from build123d import *

# Parameters (mm, degrees)
SKETCH5_R            = 22.5
BOSS_EXTRUDE4_DEPTH  = 45
SKETCH6_R            = 21
BOSS_EXTRUDE5_DEPTH  = 6
SKETCH7_R            = 22.25
BOSS_EXTRUDE6_DEPTH  = 38
SKETCH8_R            = 21
BOSS_EXTRUDE7_DEPTH  = 22
SKETCH9_R            = 18.5
BOSS_EXTRUDE9_DEPTH  = 22
CUT_EXTRUDE1_START   = -6.5
CUT_EXTRUDE1_DEPTH   = 6.5
CUT_EXTRUDE3_START   = -38
CUT_EXTRUDE3_DEPTH   = 38
BOSS_EXTRUDE11_DEPTH = 2
SKETCH19_R           = 5
BOSS_EXTRUDE12_DEPTH = 25
CUT_EXTRUDE4_DEPTH   = 10


with BuildPart() as part:
    # Sketch5 → Boss-Extrude4 (new body)
    with BuildSketch(Plane(origin=(0, 0, 0), x_dir=(1, 0, 0), z_dir=(0, 1, 0))):
        with Locations(Location((0, 0, 0), (0, 0, 90))):
            Circle(SKETCH5_R)
    extrude(amount=BOSS_EXTRUDE4_DEPTH)

    # Sketch6 → Boss-Extrude5 (add)
    with BuildSketch(Plane(origin=(0, 45, 0), x_dir=(-1, 0, 0), z_dir=(0, 1, 0))):
        with Locations(Location((0, 0, 0), (0, 0, 90))):
            Circle(SKETCH6_R)
    extrude(amount=BOSS_EXTRUDE5_DEPTH)

    # Sketch7 → Boss-Extrude6 (add)
    with BuildSketch(Plane(origin=(0, 51, 0), x_dir=(-1, 0, 0), z_dir=(0, 1, 0))):
        with Locations(Location((0, 0, 0), (0, 0, 90))):
            Circle(SKETCH7_R)
    extrude(amount=BOSS_EXTRUDE6_DEPTH)

    # Sketch8 → Boss-Extrude7 (add)
    with BuildSketch(Plane(origin=(0, 89, 0), x_dir=(-1, 0, 0), z_dir=(0, 1, 0))):
        with Locations(Location((0, 0, 0), (0, 0, 90))):
            Circle(SKETCH8_R)
    extrude(amount=BOSS_EXTRUDE7_DEPTH)

    # Sketch9 → Boss-Extrude9 (add)
    with BuildSketch(Plane(origin=(0, 111, 0), x_dir=(-1, 0, 0), z_dir=(0, 1, 0))):
        with Locations(Location((0, 0, 0), (0, 0, 90))):
            Circle(SKETCH9_R)
    extrude(amount=BOSS_EXTRUDE9_DEPTH)

    # Sketch10 → Cut-Extrude1 (cut)
    with BuildSketch(Plane(origin=(0, 133, 0), x_dir=(-1, 0, 0), z_dir=(0, 1, 0)).offset(CUT_EXTRUDE1_START)):
        with BuildLine():
            Line((-10.71607179, -15.080311847), (-4.597257497, 17.919688153))
            ThreePointArc((-4.597257497, 17.919688153), (-18.18995639, 3.372756519), (-10.71607179, -15.080311847))
        make_face()
    extrude(amount=CUT_EXTRUDE1_DEPTH, mode=Mode.SUBTRACT)

    # Sketch16 → Cut-Extrude3 (cut)
    with BuildSketch(Plane(origin=(0, 89, 0), x_dir=(1, 0, 0), z_dir=(0, 1, 0)).offset(CUT_EXTRUDE3_START)):
        with BuildLine():
            Line((0.651202062, 20.989900807), (0.68996409, 22.239299664))
            ThreePointArc((0.68996409, 22.239299664), (3.931001005, 21.899993861), (7.087715105, 21.090917348))
            Line((7.087715105, 21.090917348), (6.689528863, 19.906034351))
            ThreePointArc((6.689528863, 19.906034351), (3.710158252, 20.669657127), (0.651202062, 20.989900807))
        make_face()
    extrude(amount=CUT_EXTRUDE3_DEPTH, mode=Mode.SUBTRACT)

    # Sketch17 → Boss-Extrude11 (add)
    with BuildSketch(Plane.XZ):
        with BuildLine():
            ThreePointArc((-5, 12), (-13, 0), (-5, -12))
            Line((-5, -12), (5, -12))
            ThreePointArc((5, -12), (10.816653826, -7.211102551), (13, 0))
            ThreePointArc((13, 0), (10.816653826, 7.211102551), (5, 12))
            Line((5, 12), (-5, 12))
        make_face()
    extrude(amount=BOSS_EXTRUDE11_DEPTH)

    # Sketch19 → Boss-Extrude12 (add)
    with BuildSketch(Plane.XZ.offset(2)):
        with Locations(Location((0, 0, 0), (0, 0, 270))):
            Circle(SKETCH19_R)
    extrude(amount=BOSS_EXTRUDE12_DEPTH)

    # Sketch20 → Cut-Extrude4 (cut)
    with BuildSketch(Plane.XZ):
        with BuildLine():
            ThreePointArc((-10.577989001, 12.167341234), (-13.992202563, 13.581554796), (-12.577989001, 10.167341234))
            Line((-12.577989001, 10.167341234), (-12.577989001, 12.167341234))
            Line((-12.577989001, 12.167341234), (-10.577989001, 12.167341234))
        make_face()
        with BuildLine():
            Line((-12.577989001, 12.167341234), (-12.577989001, 10.167341234))
            ThreePointArc((-12.577989001, 10.167341234), (-11.163775438, 10.753127672), (-10.577989001, 12.167341234))
            Line((-10.577989001, 12.167341234), (-12.577989001, 12.167341234))
        make_face()
        with BuildLine():
            Line((-12.577989001, -10.167341234), (-12.577989001, -12.167341234))
            Line((-12.577989001, -12.167341234), (-10.577989001, -12.167341234))
            ThreePointArc((-10.577989001, -12.167341234), (-11.163775438, -10.753127672), (-12.577989001, -10.167341234))
        make_face()
        with BuildLine():
            Line((-10.577989001, -12.167341234), (-12.577989001, -12.167341234))
            Line((-12.577989001, -12.167341234), (-12.577989001, -10.167341234))
            ThreePointArc((-12.577989001, -10.167341234), (-13.992202563, -13.581554796), (-10.577989001, -12.167341234))
        make_face()
        with BuildLine():
            ThreePointArc((12.577989001, -10.167341234), (11.163775438, -10.753127672), (10.577989001, -12.167341234))
            Line((10.577989001, -12.167341234), (12.577989001, -12.167341234))
            Line((12.577989001, -12.167341234), (12.577989001, -10.167341234))
        make_face()
        with BuildLine():
            Line((12.577989001, -12.167341234), (10.577989001, -12.167341234))
            ThreePointArc((10.577989001, -12.167341234), (12.577989001, -14.167341234), (14.577989001, -12.167341234))
            ThreePointArc((14.577989001, -12.167341234), (13.992202563, -10.753127672), (12.577989001, -10.167341234))
            Line((12.577989001, -10.167341234), (12.577989001, -12.167341234))
        make_face()
        with BuildLine():
            ThreePointArc((10.577989001, 12.167341234), (11.163775438, 10.753127672), (12.577989001, 10.167341234))
            Line((12.577989001, 10.167341234), (12.577989001, 12.167341234))
            Line((12.577989001, 12.167341234), (10.577989001, 12.167341234))
        make_face()
        with BuildLine():
            Line((12.577989001, 12.167341234), (12.577989001, 10.167341234))
            ThreePointArc((12.577989001, 10.167341234), (13.992202563, 10.753127672), (14.577989001, 12.167341234))
            ThreePointArc((14.577989001, 12.167341234), (12.577989001, 14.167341234), (10.577989001, 12.167341234))
            Line((10.577989001, 12.167341234), (12.577989001, 12.167341234))
        make_face()
    extrude(amount=-CUT_EXTRUDE4_DEPTH, mode=Mode.SUBTRACT)


solid = part.part
Read the model definition and answer for the solid it produces. Units are mm, in the model's axes. A direction names the side the tool comes from. Round coordinates to 2 decimals unless told otherwise and drop trailing zeros. Write each loop counter-clockwise with the first axis right and the second up, starting at its lowest first coordinate (ties: lowest second). Pieces come first, ordered by that corner, then holes. Notation, with made-up numbers: (30, 59) - (42, 59) arc R8 cw to (42, 68) - close; hole circle Ø5 at (3, 42). An arc over 180 degrees is marked (long way). Use a Markdown table: item, result.
(1) Which of the six approach directions +Z, -Z, +X, -X, +Y, -Y give full straight-line access (tool end or side, diameter ignored) to faces 4 (the flat face through (-13, 10, 12)), 5 (the cylindrical face through (-13, -1, 0)), 6 (the flat face through (-19, 111, 0))?
Reported:
| item | result |
|---|---|
| face 4 | -Y |
| face 5 | -X, -Y |
| face 6 | +Y |
(2) The part is cut by section D-D (y = -14). Write down the section's boundary in (x, z).
Reported:
| item | result |
|---|---|
| outline | circle Ø10 at (0, 0) |
(3) The part is cut by section C-C (z = 16). Write down the section's boundary in (x, y), then the cut area to 3 significant figures.
Reported:
| item | result |
|---|---|
| outline | (-15.82, 0) - (15.82, 0) - (15.82, 45) - (13.6, 45) - (13.6, 51) - (15.46, 51) - (15.46, 89) - (13.6, 89) - (13.6, 111) - (9.29, 111) - (9.29, 126.5) - (4.95, 126.5) - (4.95, 133) - (-9.29, 133) - (-9.29, 111) - (-13.6, 111) - (-13.6, 89) - (-15.46, 89) - (-15.46, 51) - (-13.6, 51) - (-13.6, 45) - (-15.82, 45) - close |
| area | 3,740 mm2 |
(4) The mould has two halves that part along X. Classify faces 1 (the flat face through (7.7, 129.7, 1.19)), 2 (the flat face through (-13, 10, -12)), 3 (the cylindrical face through (-4.846, 69.734, 21.716)): released by +X, released by -X, zero draft, split by the parting line, or undercut.
Reported:
| item | result |
|---|---|
| face 1 | released by +X |
| face 2 | undercut |
| face 3 | split by the parting line |
(5) Straight lines are drawn through the part: line 1 along Y through (x, z) = (20.5, -5.5); line 2 along Y through (x, z) = (4.5, 3); line 3 along Y through (x, z) = (9.5, 13). For each, find the intervals that lie inside material, in ascending order. Write a range as [from, to].
Reported:
| item | result |
|---|---|
| line 1 | [0, 45], [51, 89] |
| line 2 | [-2, 133] |
| line 3 | [0, 126.5] |
(6) The part is cut by section B-B (x = 17). Write down the section's boundary in (y, z).
Reported:
| item | result |
|---|---|
| outline | (0, -14.74) - (45, -14.74) - (45, -12.33) - (51, -12.33) - (51, -14.35) - (89, -14.35) - (89, -12.33) - (111, -12.33) - (111, -7.3) - (126.5, -7.3) - (126.5, 7.3) - (111, 7.3) - (111, 12.33) - (89, 12.33) - (89, 14.35) - (51, 14.35) - (51, 12.33) - (45, 12.33) - (45, 14.74) - (0, 14.74) - close |
(7) The part is cut by section A-A (y = 6.5). Write down the section's boundary in (x, z), then the cut area to 3 significant figures.
Reported:
| item | result |
|---|---|
| outline | circle Ø45 at (0, 0); hole circle Ø4 at (-12.58, -12.17); hole circle Ø4 at (-12.58, 12.17); hole circle Ø4 at (12.58, -12.17); hole circle Ø4 at (12.58, 12.17) |
| area | 1,540 mm2 |
(8) Each of these flat-tipped pins is pushed along its axis until it touches: pin 1 Ø1 at (x, y) = (11, 31.5) entering from -Z; pin 2 Ø4.5 at (x, z) = (-12.5, 12.5) entering from -Y; pin 3 Ø3.5 at (x, z) = (-12.58, 12.17) entering from -Y; pin 4 Ø21 at (x, z) = (8.5, 7.5) entering from +Y. Where does it stop, or does it pass through?
Reported:
| item | result |
|---|---|
| pin 1 | z = -19.9 |
| pin 2 | y = 0 |
| pin 3 | y = 10 |
| pin 4 | y = 133 |
